from build123d import *

# Parameters (mm, degrees)
SKIZZE1_R                       = 15
AUFSATZ_LINEAR_AUSTRAGEN1_DEPTH = 3
AUFSATZ_LINEAR_START            = 2
SKIZZE2_R                       = 15
SKIZZE2_R_2                     = 13
AUFSATZ_LINEAR_AUSTRAGEN2_DEPTH = 2
AUFSATZ_LINEAR_AUSTRAGEN3_DEPTH = 1


with BuildPart() as part:
    # Skizze1 → Aufsatz-Linear austragen1 (new body)
    with BuildSketch(Plane(origin=(0, 0, 0), x_dir=(1, 0, 0), z_dir=(0, 1, 0))):
        with Locations(Location((0, 0, 0), (0, 0, 270))):
            Circle(SKIZZE1_R)
    extrude(amount=-AUFSATZ_LINEAR_AUSTRAGEN1_DEPTH)

    # Skizze2 → Aufsatz-Linear austragen2 (add)
    with BuildSketch(Plane(origin=(0, 0, 0), x_dir=(1, 0, 0), z_dir=(0, 1, 0)).offset(AUFSATZ_LINEAR_START)):
        with Locations(Location((0, 0, 0), (0, 0, 270))):
            Circle(SKIZZE2_R)
        with Locations(Location((0, 0, 0), (0, 0, 270))):
            Circle(SKIZZE2_R_2, mode=Mode.SUBTRACT)
    extrude(amount=-AUFSATZ_LINEAR_AUSTRAGEN2_DEPTH)

    # Skizze3 → Aufsatz-Linear austragen3 (add)
    with BuildSketch(Plane(origin=(0, 2, 0), x_dir=(1, 0, 0), z_dir=(0, 1, 0))):
        with BuildLine():
            Line((-6.042078394, -7.968267609), (-7.854701912, -10.358747891))
            ThreePointArc((-7.854701912, -10.358747891), (-12.566291217, -3.329913671), (-11.953670509, 5.109771166))
            Line((-11.953670509, 5.109771166), (-9.195131161, 3.930593205))
            ThreePointArc((-9.195131161, 3.930593205), (-9.666377859, -2.561472055), (-6.042078394, -7.968267609))
        make_face()
        with BuildLine():
            Line((6.042078394, 7.968267609), (7.854701912, 10.358747891))
            ThreePointArc((7.854701912, 10.358747891), (12.566291217, 3.329913671), (11.953670509, -5.109771166))
            Line((11.953670509, -5.109771166), (9.195131161, -3.930593205))
            ThreePointArc((9.195131161, -3.930593205), (9.666377859, 2.561472055), (6.042078394, 7.968267609))
        make_face()
    extrude(amount=-AUFSATZ_LINEAR_AUSTRAGEN3_DEPTH)


solid = part.part
Work out the finished part from the listing and answer in its coordinate system (mm). A direction names the side the tool comes from. Coordinates: 2 decimals unless noted, no trailing zeros. Write each loop counter-clockwise with the first axis right and the second up, starting at its lowest first coordinate (ties: lowest second). Pieces come first, ordered by that corner, then holes.
1. The part is cut by section D-D, the plane x = 6.5. Write down the section's boundary in (y, z), and give its area (3 significant figures).
Results list:
outline: (-3, -13.52) - (2, -13.52) - (2, -11.26) - (0, -11.26) - (0, 11.26) - (2, 11.26) - (2, 13.52) - (-3, 13.52) - close; (1, -8.57) - (2, -8.57) - (2, -7.6) - (1, -7.6) - close
area: 91.1 mm2
2. The part is cut by section C-C, the plane y = -1.65. Write down the section's boundary in (x, z), and give its area (3 significant figures).
Results list:
outline: circle Ø30 at (0, 0)
area: 707 mm2
3. For faces 5 (the flat face through (10.594, 1.507, 4.528)), 6 (the flat face through (0, -3, 0)), 7 (the flat face through (10, 1, -3)), determine the directions among +Z, -Z, +X, -X, +Y, -Y from which every point of the face is accessible in a straight line to the end or side of a thin tool.
Results list:
face 5: +Y
face 6: +Z, -Z, +X, -X, -Y
face 7: none
4. For a pull along Z with two mould halves and no side action, classify faces 1 (the flat face through (9, 2, -5)), 2 (the cylindrical face through (0.66, -0.465, -14.985)), 3 (the flat face through (0, 0, 0)), 4 (the cylindrical face through (3.9, 0.8, 12.4)) as +Z half, -Z half, draft (parallel to the pull), parting line (faces both ways), or undercut.
Results list:
face 1: draft
face 2: parting line
face 3: undercut
face 4: undercut
5. The part is cut by section B-B, the plane z = 0. Write down the section's boundary in (x, y).
Results list:
outline: (-15, -3) - (15, -3) - (15, 2) - (10, 2) - (10, 1) - (13, 1) - (13, 0) - (-13, 0) - (-13, 1) - (-10, 1) - (-10, 2) - (-15, 2) - close
6. The part is cut by section A-A, the plane x = 0. Write down the section's boundary in (y, z), and give its area (3 significant figures).
Results list:
outline: (-3, -15) - (2, -15) - (2, -13) - (0, -13) - (0, 13) - (2, 13) - (2, 15) - (-3, 15) - close
area: 98.0 mm2
7. Flat-ended cylindrical pins translate along their axes: pin 1 (3 mm diameter, centred on x = -10, y = -0.5, fed in from -Z); pin 2 (1.5 mm diameter, centred on x = -7.5, y = -0.5, fed in from -Z); pin 3 (2 mm diameter, centred on y = -2.5, z = -11, fed in from -X). Find the tip coordinate at first contact, or state that the pin passes through.
Results list:
pin 1: stops at z = -12.36
pin 2: stops at z = -13.4
pin 3: stops at x = -11.18
8. Consider line 1 along X through (y, z) = (0.1, 0.25); line 2 along X through (y, z) = (1.4, 0); line 3 along Y through (x, z) = (11, 1.5). Determine where each line is inside the solid, lowest interval first.
Results list:
line 1: x = -15 to -13, 13 to 15
line 2: x = -15 to -10, 10 to 15
line 3: y = -3 to 0, 1 to 2
